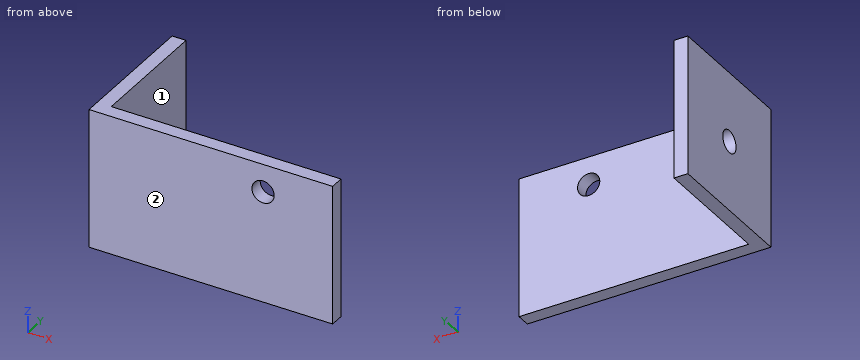
```python
from build123d import *

# Parameters (mm, degrees)
EXTRUDE_1_DEPTH     = 20
SKETCH_3_R          = 1.6
CUT_EXTRUDE_2_DEPTH = 36
SKETCH_4_R          = 1.6
CUT_EXTRUDE_3_DEPTH = 21


with BuildPart() as part:
    # Эскиз1 → Бобышка-Вытянуть1 (new body)
    with BuildSketch(Plane.XY):
        Polygon((0, 0), (35, 0), (35, 2), (2, 2), (2, 20), (0, 20), align=None)
    extrude(amount=EXTRUDE_1_DEPTH)

    # Эскиз3 → Вырез-Вытянуть2 (cut, through all)
    with BuildSketch(Plane.ZY):
        with Locations((10, 10)):
            Circle(SKETCH_3_R)
    extrude(amount=-CUT_EXTRUDE_2_DEPTH, mode=Mode.SUBTRACT)

    # Эскиз4 → Вырез-Вытянуть3 (cut, through all)
    with BuildSketch(Plane.XZ):
        with Locations((25, 16)):
            Circle(SKETCH_4_R)
    extrude(amount=-CUT_EXTRUDE_3_DEPTH, mode=Mode.SUBTRACT)


solid = part.part
```
Model file for the job. Use its own axes, mm. Face numbers are marked on the shaded views. A direction names the side the tool comes from. Coordinates: 2 decimals unless noted, no trailing zeros. Order: outer loops, then holes, each group sorted by start corner. A loop starts at its lowest first (then second) coordinate and runs counter-clockwise, first axis right, second up. Notation, with made-up numbers: (35.5, -36) -> (44.5, -36) arc R11 cw to (44.5, -20) -> close; hole circle Ø5 at (82.25, 67). An arc over 180 degrees is marked (long way). Answer as a JSON object with one key per item and string values. Group by question number.
1) Cut at B-B, the plane y = 10. Write the cut outline in (x, z), then the cut area to 3 significant figures.
2) Flat gauge pins, fed straight in: pin 1 (3 mm diameter, centred on y = 13, z = 9, fed in from +X); pin 2 (10 mm diameter, centred on x = 20.5, z = 9, fed in from +Y). Where does each tip first touch, or does it go through?
3) Cut at D-D, the plane y = 3.25. Write the cut outline in (x, z), then the cut area to 3 significant figures.
4) Which spindle directions (+Z, -Z, +X, -X, +Y, -Y) get a long thin tool onto all of the face, cutting with end or side? Do the marked faces 1 and 2. Say none if no direction does.
5) Cut at C-C, the plane z = 10. Write the cut outline in (x, y), then the cut area to 3 significant figures.
6) Cut at A-A, the plane x = 25. Write the cut outline in (y, z).
7) Drill centre lines: L1, parallel to Y at x = 0.75, z = 10; L2, parallel to Z at x = 25, y = 0.65; L3, parallel to X at y = 6.75, z = 16. Where is each one in solid material? Low to high.
Check values:
{
 "1": {"outline": "(0, 0) -> (2, 0) -> (2, 8.4) -> (0, 8.4) -> close; (0, 11.6) -> (2, 11.6) -> (2, 20) -> (0, 20) -> close", "area": "33.6 mm²"},
 "2": {"pin 1": "stops at x = 2", "pin 2": "stops at y = 2"},
 "3": {"outline": "(0, 0) -> (2, 0) -> (2, 20) -> (0, 20) -> close", "area": "40.0 mm²"},
 "4": {"face 1": "+Z, -Z, +X, +Y", "face 2": "+Z, -Z, +X, -X, -Y"},
 "5": {"outline": "(0, 0) -> (35, 0) -> (35, 2) -> (2, 2) -> (2, 8.4) -> (0, 8.4) -> close; (0, 11.6) -> (2, 11.6) -> (2, 20) -> (0, 20) -> close", "area": "99.6 mm²"},
 "6": {"outline": "(0, 0) -> (2, 0) -> (2, 14.4) -> (0, 14.4) -> close; (0, 17.6) -> (2, 17.6) -> (2, 20) -> (0, 20) -> close"},
 "7": {"L1": "y = 0 to 8.4, 11.6 to 20", "L2": "z = 0 to 14.4, 17.6 to 20", "L3": "x = 0 to 2"}
}
